Geometry: final body of the model. Coordinates: model frame, mm. A direction names the side the tool comes from. Round coordinates to 2 decimals unless told otherwise and drop trailing zeros. Order: outer loops, then holes, each group sorted by start corner. A loop starts at its lowest first (then second) coordinate and runs counter-clockwise, first axis right, second up. Notation, with made-up numbers: (45, 10) -> (91, 10) arc R7 cw to (91, 22) -> close; hole circle Ø3 at (-35.5, 25.25). An arc over 180 degrees is marked (long way). Put each result on its own line as item: value.
```python
from build123d import *

# Parameters (mm, degrees)
F0_W     = 10
F0_H     = 202
F1_DEPTH = 25


with BuildPart() as f1:
    # F0 (on Right) → F1 (new body)
    with BuildSketch(Plane.YZ):
        Polygon((183, 151.398099), (198, 151.398099), (198, 161.398099), (-198, 161.398099), (-198, 151.398099), (-183, 151.398099), (-173, 151.398099), (173, 151.398099), align=None)
        with Locations((-178, 50.398099)):
            Rectangle(F0_W, F0_H)
        Polygon((183, -60.601901), (183, -50.601901), (173, -50.601901), (-173, -50.601901), (-183, -50.601901), (-183, -60.601901), align=None)
        with Locations((178, 50.398099)):
            Rectangle(F0_W, F0_H)
    extrude(amount=F1_DEPTH)


solid = f1.part
```
1. Contact query for flat-ended pins moving along their axis: P1, Ø8, axis at x = 4.5, z = 7, coming from the -Y side; P2, Ø12.5, axis at x = 8.5, z = 18.5, coming from the +Y side; P3, Ø7.5, axis at x = 14.5, y = 189, coming from the -Z side. Output: stop coordinate, or through.
Ans:
P1: y = -183
P2: y = 183
P3: z = 151.4
2. Cut plane A-A on y = 69.5. Return loops of the section in (x, z).
Ans:
outline: (0, -60.6) -> (25, -60.6) -> (25, -50.6) -> (0, -50.6) -> close; (0, 151.4) -> (25, 151.4) -> (25, 161.4) -> (0, 161.4) -> close
3. Cut plane B-B on z = 60.5. Return loops of the section in (x, y), and give its area (3 significant figures).
Ans:
outline: (0, -183) -> (25, -183) -> (25, -173) -> (0, -173) -> close; (0, 173) -> (25, 173) -> (25, 183) -> (0, 183) -> close
area: 500 mm²
4. Set-up query: faces 1 (the face through (12, 2, -50.602)), 2 (the face through (12, 190, 151.398)), 3 (the face through (12, -191, 151.398)). Return all of +Z, -Z, +X, -X, +Y, -Y with unobstructed straight access to the full face (end or side cutting, diameter ignored); none if empty.
Ans:
face 1: +X, -X
face 2: -Z, +X, -X, +Y
face 3: -Z, +X, -X, -Y
5. Cut plane C-C on x = 13. Return loops of the section in (y, z), and give its area (3 significant figures).
Ans:
outline: (-198, 151.4) -> (-183, 151.4) -> (-183, -60.6) -> (183, -60.6) -> (183, 151.4) -> (198, 151.4) -> (198, 161.4) -> (-198, 161.4) -> close; hole (-173, -50.6) -> (173, -50.6) -> (173, 151.4) -> (-173, 151.4) -> close
area: 11,700 mm²
6. Draft query along Y for faces 4 (the face through (0, -1, 158)), 5 (the face through (12, -183, 47)), 6 (the face through (12, -173, 49)). Return one class per face: +Y half, -Y half, draft (parallel to the pull), parting line (faces both ways), or undercut.
Ans:
face 4: draft
face 5: -Y half
face 6: undercut
7. Material intervals for probe 1 along Y at (x, z) = (6.5, -22.5); probe 2 along Z at (x, y) = (8, -97), sorted ascending.
Ans:
probe 1: -183 to -173, 173 to 183
probe 2: -60.6 to -50.6, 151.4 to 161.4
